```python
from build123d import *

# Parameters (mm, degrees)
F1_DEPTH = 314.325
F2_R     = 4.7625
F3_DEPTH = 50.801
F4_R     = 4.7625
F5_DEPTH = 6.351


with BuildPart() as f1:
    # F0 (on Right) → F1 (new body, symmetric)
    with BuildSketch(Plane.YZ):
        Polygon((0, 44.45), (0, 0), (6.35, 0), (6.35, 50.8), (-44.45, 50.8), (-44.45, 44.45), align=None)
    extrude(amount=F1_DEPTH, both=True)

    # F2 (on face) → F3 (cut, through all)
    with BuildSketch(Plane(origin=(0, 6.35, 0), x_dir=(-1, 0, 0), z_dir=(0, 1, 0))):
        with Locations((-19.05, 25.4)):
            Circle(F2_R)
        with Locations((19.05, 25.4)):
            Circle(F2_R)
    extrude(amount=-F3_DEPTH, mode=Mode.SUBTRACT)

    # F4 (on face) → F5 (cut, through all)
    with BuildSketch(Plane(origin=(0, 0, 44.45), x_dir=(1, 0, 0), z_dir=(0, 0, -1))):
        with Locations((-298.45, 19.05)):
            Circle(F4_R)
        with Locations((298.45, 19.05)):
            Circle(F4_R)
    extrude(amount=-F5_DEPTH, mode=Mode.SUBTRACT)


solid = f1.part
```
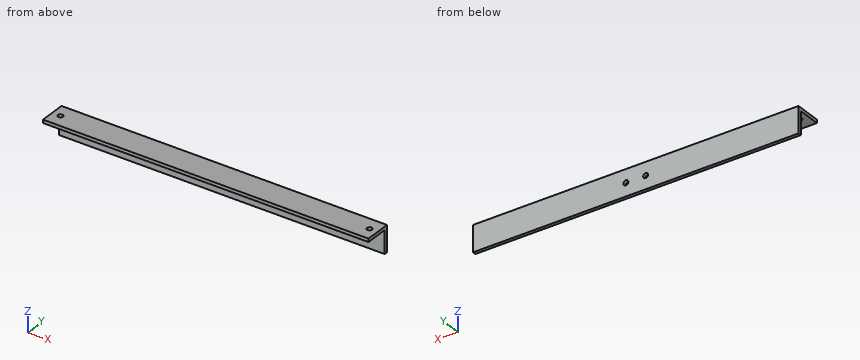
Input: part model. Units: mm. Frame: model coordinates. Give positions to 0.01 mm unless a question says otherwise; leave off trailing zeros. Order: outer loops, then holes, each group sorted by start corner. A loop starts at its lowest first (then second) coordinate and runs counter-clockwise, first axis right, second up. Notation, with made-up numbers: M 46,60.25 L 70,60.25 A22 cw 70,81.25 Z; hole C 36,-23 d10. An arc over 180 degrees is marked long. One line per question, with ' | ' between items. Start each with the question number.
1. First-contact query: pin 1 Ø22 at (x, z) = (9, 26) entering from -Y; pin 2 Ø5 at (x, y) = (-250, -8) entering from -Z; pin 3 Ø8.5 at (x, z) = (19.05, 25.4) entering from +Y. Flat tips, straight axial feed; report the tip coordinate or a pass-through.
2. Section query A-A (x = 166.5). Return the cut outline in (y, z), and give its area (3 significant figures).
3. Section query B-B (y = -7). Return the cut outline in (x, z) (3 decimals), and give its area (3 significant figures).
4. Material intervals for probe 1 along X at (y, z) = (-19.05, 49) (1 decimal); probe 2 along Z at (x, y) = (-19.05, 5); probe 3 along Y at (x, z) = (298.45, 46), sorted ascending. Write a range as [from, to].
Here are the results:
1) pin 1: y = 0 | pin 2: z = 44.45 | pin 3: through
2) outline: M -44.45,44.45 L 0,44.45 L 0,0 L 6.35,0 L 6.35,50.8 L -44.45,50.8 Z | area: 605 mm²
3) outline: M -314.325,44.45 L 314.325,44.45 L 314.325,50.8 L -314.325,50.8 Z | area: 3,990 mm²
4) probe 1: [-314.3, -303.2], [-293.7, 293.7], [303.2, 314.3] | probe 2: [0, 20.64], [30.16, 50.8] | probe 3: [-44.45, -23.81], [-14.29, 6.35]
